from build123d import *

# Parameters (mm, degrees)
F1_DEPTH  = 50
F3_DEPTH  = 25
F4_W      = 68
F4_H      = 45
F4_R      = 6
F5_DEPTH  = 13
F6_R      = 3
F8_DEPTH  = 32
F9_R      = 6
F10_DEPTH = 25


with BuildPart() as f1:
    # F0 (on Front) → F1 (new body, symmetric)
    with BuildSketch(Plane.XZ):
        Polygon((-32, 25), (-32, 0), (-10, 0), (-10, 6), (-19, 6), (-19, 12), (19, 12), (19, 6), (10, 6), (10, 0), (32, 0), (32, 25), align=None)
    extrude(amount=F1_DEPTH, both=True)

    # F2 (on face) → F3 (join)
    with BuildSketch(Plane.YZ.offset(32)):
        Polygon((50, 0), (50, 25), (50, 70), (14, 70), (14, 42), (-18, 42), (-18, 25), (-18, 0), align=None)
    extrude(amount=-F3_DEPTH)

    # F4 (on face) → F5 (join)
    with BuildSketch(Plane(origin=(7, 0, 0), x_dir=(0, -1, 0), z_dir=(-1, 0, 0))):
        with Locations((-16, 47.5)):
            Rectangle(F4_W, F4_H)
        with Locations((2, 58)):
            Circle(F4_R, mode=Mode.SUBTRACT)
    extrude(amount=F5_DEPTH)

    # F6
    f6_edges = [f1.edges().sort_by_distance(p)[0] for p in [
        (0.5, -18, 70),
    ]]
    fillet(f6_edges, radius=F6_R)

    # F7 (on face) → F8 (join)
    with BuildSketch(Plane.XZ.offset(50)):
        with BuildLine():
            Line((6, 25), (20, 25))
            ThreePointArc((20, 25), (0, 45), (-20, 25))
            Line((-20, 25), (-6, 25))
            ThreePointArc((-6, 25), (0, 31), (6, 25))
        make_face()
        with BuildLine():
            Line((-6, 25), (6, 25))
            ThreePointArc((6, 25), (0, 31), (-6, 25))
        make_face()
        with BuildLine():
            ThreePointArc((-6, 25), (0, 19), (6, 25))
            Line((6, 25), (-6, 25))
        make_face()
    extrude(amount=-F8_DEPTH)

    # F9 (on face) → F10 (cut)
    with BuildSketch(Plane.XZ.offset(50)):
        with Locations((0, 25)):
            Circle(F9_R)
    extrude(amount=-F10_DEPTH, mode=Mode.SUBTRACT)


solid = f1.part
Verification items for the finished model (mm, model axes). A direction names the side the tool comes from. Coordinates: 2 decimals unless noted, no trailing zeros. Order: outer loops, then holes, each group sorted by start corner. A loop starts at its lowest first (then second) coordinate and runs counter-clockwise, first axis right, second up.
Item 1: Release check for a two-part mould opening along X. For faces 4 (the face through (-14, -1, 6)), 5 (the face through (-12, -18, 33)), 6 (the face through (-32, -1, 13)) record: +X half, -X half, draft (parallel to the pull), parting line (faces both ways), or undercut.
Filled in:
face 4: undercut
face 5: draft
face 6: -X half
Item 2: Section check C-C, the plane x = 0. Enter the section's corners in (y, z).
Filled in:
outline: (-50, 12) - (50, 12) - (50, 70) - (-15, 70) arc R3 ccw to (-18, 67) - (-18, 45) - (-50, 45) - (-50, 31) - (-25, 31) - (-25, 19) - (-50, 19) - close; hole circle Ø12 at (-2, 58)
Item 3: Section check D-D, the plane y = 11. Enter the section's corners in (x, z).
Filled in:
outline: (-32, 0) - (-10, 0) - (-10, 6) - (-19, 6) - (-19, 12) - (7, 12) - (7, 0) - (32, 0) - (32, 42) - (7, 42) - (7, 70) - (-6, 70) - (-6, 25) - (-32, 25) - close
Item 4: Section check A-A, the plane z = 58. Enter the section's corners in (x, y).
Filled in:
outline: (-6, -18) - (7, -18) - (7, -8) - (-6, -8) - close; (-6, 4) - (7, 4) - (7, 14) - (32, 14) - (32, 50) - (-6, 50) - close
Item 5: Material ranges on L1, parallel to Z at x = 0, y = -33; L2, parallel to Z at x = -15.5, y = 4; L3, parallel to X at y = 43, z = 10, recorded low to high.
Filled in:
L1: z = 12 to 19, 31 to 45
L2: z = 0 to 6, 12 to 25
L3: x = -32 to -19, 7 to 32
Item 6: Access from +Z, -Z, +X, -X, +Y, -Y to the whole of each face (thin tool, end or side, straight path). Record for faces 1 (the face through (-19, -1, 9)), 2 (the face through (10, -34, 3)), 3 (the face through (26, -34, 25)).
Filled in:
face 1: +Y, -Y
face 2: -Z, -Y
face 3: +Z, +X, -Y
Item 7: Depth check by flat-ended pin: pin 1 (4 mm diameter, centred on x = -11.5, z = 38.5, fed in from +Y); pin 2 (10 mm diameter, centred on y = 33.5, z = 38.5, fed in from -X); pin 3 (3.5 mm diameter, centred on x = 29, y = -28, fed in from +Z); pin 4 (9.5 mm diameter, centred on y = -2, z = 58, fed in from -X). Enter the tip coordinate at first touch or a pass-through.
Filled in:
pin 1: stops at y = -18
pin 2: stops at x = -6
pin 3: stops at z = 25
pin 4: passes through
Item 8: Section check B-B, the plane y = -2. Enter the section's corners in (x, z).
Filled in:
outline: (-32, 0) - (-10, 0) - (-10, 6) - (-19, 6) - (-19, 12) - (7, 12) - (7, 0) - (32, 0) - (32, 42) - (7, 42) - (7, 52) - (-6, 52) - (-6, 25) - (-32, 25) - close; (-6, 64) - (7, 64) - (7, 70) - (-6, 70) - close
